For this review, take the finished solid that the model builds, in its own axes (mm). Face numbers are marked on the shaded views. A direction names the side the tool comes from. Give positions to 0.01 mm unless a question says otherwise; leave off trailing zeros. Write each loop counter-clockwise with the first axis right and the second up, starting at its lowest first coordinate (ties: lowest second). Pieces come first, ordered by that corner, then holes.
Q1. Machinability: for the marked faces 4, 5 and 6, which of the approach directions +Z, -Z, +X, -X, +Y, -Y give a long, thin tool a straight path to every point of the face, cutting with its end or side? Answer none if there is none.
Q2. We need section C-C (z = -5.75). Write out the cut boundary in (x, y), then the cut area to 3 significant figures.
Q3. We need section B-B (z = -11.5). Write out the cut boundary in (x, y).
Q4. We need section A-A (x = 19.5). Write out the cut boundary in (y, z) (3 decimals), then the cut area to 3 significant figures.
Q5. Insertion check: P1, Ø5, axis at y = 9, z = -6, coming from the -X side; P2, Ø1.6, axis at y = 4, z = -1, coming from the +X side; P3, Ø4.5, axis at x = 38.1, z = -6.604, coming from the -Y side; P4, Ø6.5, axis at x = 39, z = -6, coming from the +Y side. Each pin has a flat end and moves straight along its axis. Give the tip position at first contact, or say it passes through.
Q6. For line 1 (Z direction, x = 38, y = 52); line 2 (Y direction, x = 36.5, z = -12); line 3 (Z direction, x = 20.5, y = 12) (3 decimals), list the stretches that pass through material, from the lowest coordinate up.
Q7. We need section D-D (x = 25.5). Write out the cut boundary in (y, z) (3 decimals).
Q8. Mouldability with a two-part tool opening along Y and no side actions: class the marked faces 1, 2 and 3 as released by +Y, released by -Y, zero draft, split by the parting line, or undercut.
```python
from build123d import *

# Parameters (mm, degrees)
SKETCH1_W           = 29.591
SKETCH1_H           = 3.175
SKETCH1_R           = 6.604
BOSS_EXTRUDE1_DEPTH = 76.2
SKETCH2_R           = 4.191
CUT_EXTRUDE1_DEPTH  = 50.8
SKETCH1_3_R         = 6.604
CUT_EXTRUDE2_DEPTH  = 8.89
CUT_EXTRUDE3_START  = 27.94
SKETCH1_5_R         = 6.604
CUT_EXTRUDE3_DEPTH  = 17.78
SKETCH3_R           = 2.54
CUT_EXTRUDE4_DEPTH  = 90.327145258
CUT_EXTRUDE5_START  = 67.31
SKETCH1_6_R         = 6.604
CUT_EXTRUDE5_DEPTH  = 8.89
FILLET1_R           = 7.62
FILLET2_R           = 7.62


with BuildPart() as part:
    # Sketch1 → Boss-Extrude1 (new body)
    with BuildSketch(Plane(origin=(0, 0, 0), x_dir=(1, 0, 0), z_dir=(0, 1, 0))):
        with Locations((14.7955, 1.5875)):
            Rectangle(SKETCH1_W, SKETCH1_H)
        with BuildLine():
            Line((32.455996545, 3.175), (29.591, 3.175))
            Line((29.591, 3.175), (29.591, 0))
            Line((29.591, 0), (38.1, 0))
            ThreePointArc((38.1, 0), (34.862122609, 0.84822325), (32.455996545, 3.175))
        make_face()
        with Locations((38.1, 6.604)):
            Circle(SKETCH1_R)
    extrude(amount=BOSS_EXTRUDE1_DEPTH)

    # Sketch2 → Cut-Extrude1 (cut)
    with BuildSketch(Plane(origin=(0, 0, -3.175), x_dir=(-1, 0, 0), z_dir=(0, 0, -1))):
        with Locations((-19.431, 56.769)):
            Circle(SKETCH2_R)
        with Locations((-19.431, 19.431)):
            Circle(SKETCH2_R)
    extrude(amount=-CUT_EXTRUDE1_DEPTH, mode=Mode.SUBTRACT)

    # Sketch1_3 → Cut-Extrude2 (cut)
    with BuildSketch(Plane(origin=(0, 0, 0), x_dir=(1, 0, 0), z_dir=(0, 1, 0))):
        with BuildLine():
            Line((32.455996545, 3.175), (29.591, 3.175))
            Line((29.591, 3.175), (29.591, 0))
            Line((29.591, 0), (38.1, 0))
            ThreePointArc((38.1, 0), (34.862122609, 0.84822325), (32.455996545, 3.175))
        make_face()
        with Locations((38.1, 6.604)):
            Circle(SKETCH1_3_R)
    extrude(amount=CUT_EXTRUDE2_DEPTH, mode=Mode.SUBTRACT)

    # Sketch1_5 → Cut-Extrude3 (cut)
    with BuildSketch(Plane(origin=(0, 0, 0), x_dir=(1, 0, 0), z_dir=(0, 1, 0)).offset(CUT_EXTRUDE3_START)):
        with Locations((38.1, 6.604)):
            Circle(SKETCH1_5_R)
        with BuildLine():
            Line((32.455996545, 3.175), (29.591, 3.175))
            Line((29.591, 3.175), (29.591, 0))
            Line((29.591, 0), (38.1, 0))
            ThreePointArc((38.1, 0), (34.862122609, 0.84822325), (32.455996545, 3.175))
        make_face()
    extrude(amount=CUT_EXTRUDE3_DEPTH, mode=Mode.SUBTRACT)

    # Sketch3 → Cut-Extrude4 (cut, through all)
    with BuildSketch(Plane(origin=(0, 76.2, 0), x_dir=(1, 0, 0), z_dir=(0, 1, 0))):
        with Locations(Location((38.1, 6.604, 0), (0, 0, 270))):
            Circle(SKETCH3_R)
    extrude(amount=-CUT_EXTRUDE4_DEPTH, mode=Mode.SUBTRACT)

    # Sketch1_6 → Cut-Extrude5 (cut)
    with BuildSketch(Plane(origin=(0, 0, 0), x_dir=(1, 0, 0), z_dir=(0, 1, 0)).offset(CUT_EXTRUDE5_START)):
        with Locations((38.1, 6.604)):
            Circle(SKETCH1_6_R)
        with BuildLine():
            Line((32.455996545, 3.175), (29.591, 3.175))
            Line((29.591, 3.175), (29.591, 0))
            Line((29.591, 0), (38.1, 0))
            ThreePointArc((38.1, 0), (34.862122609, 0.84822325), (32.455996545, 3.175))
        make_face()
    extrude(amount=CUT_EXTRUDE5_DEPTH, mode=Mode.SUBTRACT)

    # Fillet1
    fillet1_edges = [part.edges().sort_by_distance(p)[0] for p in [
        (0, 0, -1.5875),
    ]]
    fillet(fillet1_edges, radius=FILLET1_R)

    # Fillet2
    fillet2_edges = [part.edges().sort_by_distance(p)[0] for p in [
        (0, 76.2, -1.5875),
    ]]
    fillet(fillet2_edges, radius=FILLET2_R)


solid = part.part
```
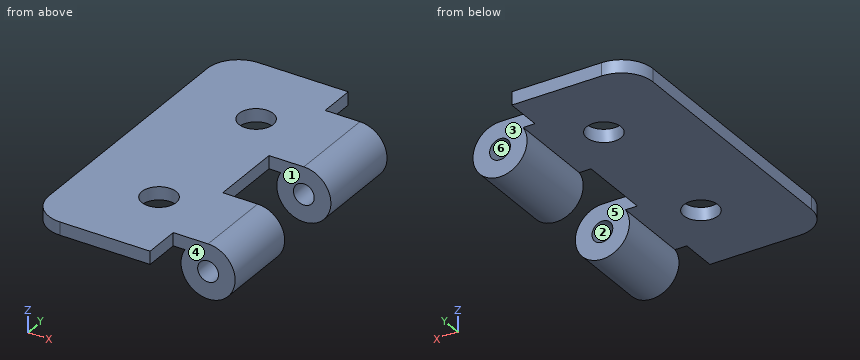
Computed:
1. face 4: +Z, -Z, +X, -Y
1. face 5: +Z, -Z, +X
1. face 6: +Y, -Y
2. outline: (31.55, 8.89) - (35.71, 8.89) - (35.71, 27.94) - (31.55, 27.94) - close; (31.55, 45.72) - (35.71, 45.72) - (35.71, 67.31) - (31.55, 67.31) - close; (40.49, 8.89) - (44.65, 8.89) - (44.65, 27.94) - (40.49, 27.94) - close; (40.49, 45.72) - (44.65, 45.72) - (44.65, 67.31) - (40.49, 67.31) - close
2. area: 338 mm2
3. outline: (33.67, 8.89) - (42.53, 8.89) - (42.53, 27.94) - (33.67, 27.94) - close; (33.67, 45.72) - (42.53, 45.72) - (42.53, 67.31) - (33.67, 67.31) - close
4. outline: (0, -3.175) - (15.241, -3.175) - (15.241, 0) - (0, 0) - close; (23.621, -3.175) - (52.579, -3.175) - (52.579, 0) - (23.621, 0) - close; (60.959, -3.175) - (76.2, -3.175) - (76.2, 0) - (60.959, 0) - close
4. area: 189 mm2
5. P1: stops at x = 31.5
5. P2: stops at x = 29.59
5. P3: passes through
5. P4: stops at y = 67.31
6. line 1: z = -13.21 to -9.14, -4.07 to 0
6. line 2: y = 8.89 to 27.94, 45.72 to 67.31
6. line 3: z = -3.175 to 0
7. outline: (0, -3.175) - (76.2, -3.175) - (76.2, 0) - (0, 0) - close
8. face 1: undercut
8. face 2: zero draft
8. face 3: released by +Y
